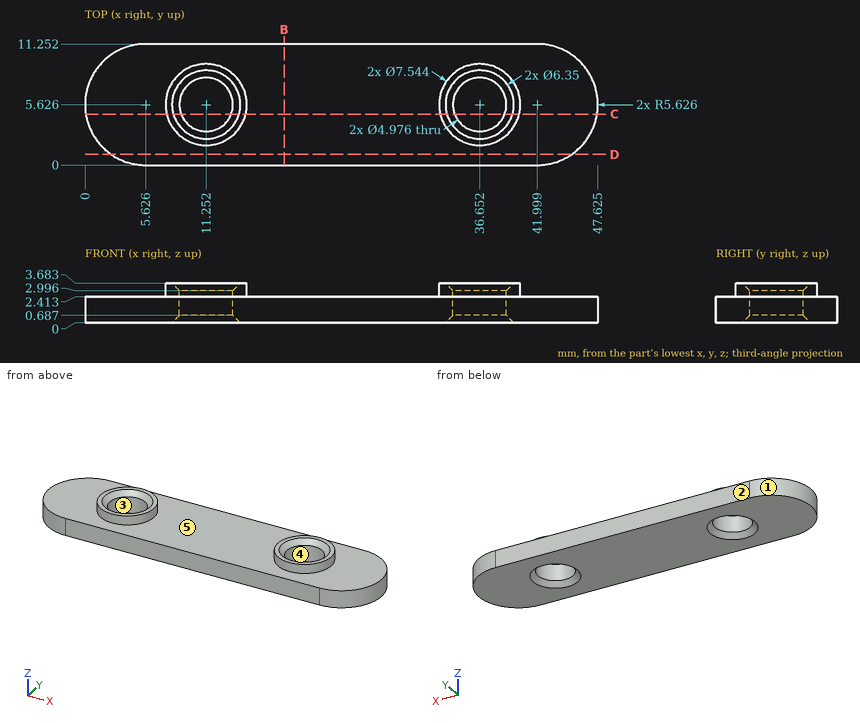
Verification items for this drawing (mm, ordinates from the low corner). A direction names the side the tool comes from. Coordinates: 2 decimals unless noted, no trailing zeros. Loops run counter-clockwise (first coordinate to the right, second up) from the corner with the lowest first, then second, coordinate; pieces in that order, holes last. Notation, with made-up numbers: (55.5, -8) -> (65.5, -8) arc R31 ccw to (65.5, 18) -> close; hole circle Ø6 at (-4.75, 42.5). An arc over 180 degrees is marked (long way). Answer in a Markdown table with one row per item. Add a question column.
1. Draft check along X on the marked faces 1, 2 and 3. Enter one of: +X half, -X half, draft (parallel to the pull), parting line (faces both ways), or undercut.
2. Section check B-B, the plane x = 18.5. Enter the section's corners in (y, z).
3. Material ranges on probe 1 along X at (y, z) = (6, 1.65); probe 2 along X at (y, z) = (4.5, 1.45); probe 3 along X at (y, z) = (4.25, 2.9) (1 decimal), recorded low to high. Write a range as [from, to].
4. Section check D-D, the plane y = 1. Enter the section's corners in (x, z), then the cut area to 3 significant figures.
5. Section check C-C, the plane y = 4.75. Give the number of separate pieces and of enclosed holes in the cut face.
6. Depth check by flat-ended pin: P1, Ø5.5, axis at x = 11.25, y = 5.63, coming from the +Z side; P2, Ø1, axis at y = 7, z = 2, coming from the +X side; P3, Ø6, axis at x = 30, y = 4, coming from the +Z side. Enter the tip coordinate at first touch or a pass-through.
7. Access from +Z, -Z, +X, -X, +Y, -Y to the whole of each face (thin tool, end or side, straight path). Record for the marked faces 4 and 5.
Derived:
| question | item | result |
|---|---|---|
| 1 | face 1 | -X half |
| 1 | face 2 | draft |
| 1 | face 3 | undercut |
| 2 | outline | (0, 0) -> (11.25, 0) -> (11.25, 2.41) -> (0, 2.41) -> close |
| 3 | probe 1 | x = [0.01, 8.79], [13.71, 34.19], [39.11, 47.61] |
| 3 | probe 2 | x = [0.11, 9.03], [13.47, 34.43], [38.87, 47.51] |
| 3 | probe 3 | x = [7.7, 9.2], [13.3, 14.8], [33.1, 34.6], [38.7, 40.2] |
| 4 | outline | (2.42, 0) -> (45.2, 0) -> (45.2, 2.41) -> (2.42, 2.41) -> close |
| 4 | area | 103 mm² |
| 5 | separate pieces | 3 |
| 5 | enclosed holes | 0 |
| 6 | P1 | stops at z = 3.26 |
| 6 | P2 | stops at x = 47.56 |
| 6 | P3 | stops at z = 2.41 |
| 7 | face 4 | +Z, -Z |
| 7 | face 5 | +Z |
